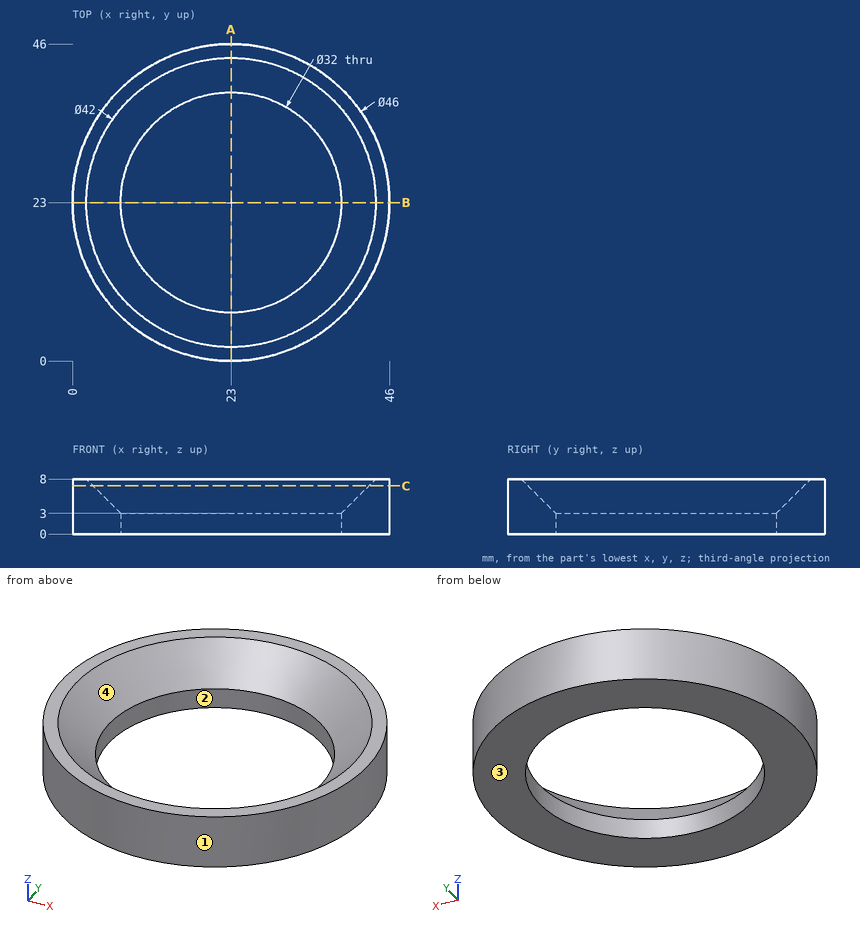
Part print with two shaded views. Sizes in mm from the minimum x, y, z corner. Coordinates: 2 decimals unless noted, no trailing zeros. Write each loop counter-clockwise with the first axis right and the second up, starting at its lowest first coordinate (ties: lowest second). Pieces come first, ordered by that corner, then holes. Notation, with made-up numbers: (58, 22) -> (62, 22) arc R20 cw to (62, 48) -> close; hole circle Ø3 at (89, -11.75). An arc over 180 degrees is marked (long way). Return JSON: item names as keys, results as strings. Group by question number.
Q1. Pull direction Y, two halves, no side cores. Call the marked faces 1, 2, 3 and 4: released by +Y, released by -Y, zero draft, split by the parting line, or undercut.
Q2. Cut at C-C, the plane z = 7. Give the cut face in (x, y).
Q3. Cut at A-A, the plane x = 23. Give the cut face in (y, z), then the cut area to 3 significant figures.
Q4. Flat gauge pins, fed straight in: pin 1 (5 mm diameter, centred on x = 37, y = 14, fed in from -Z); pin 2 (2 mm diameter, centred on x = 27, z = 5.5, fed in from -Y); pin 3 (3 mm diameter, centred on y = 25, z = 4, fed in from -X); pin 4 (3 mm diameter, centred on x = 20, z = 7, fed in from -Y). Where does each tip first touch, or does it go through?
Q5. Drill centre lines: line 1 (X direction, y = 23, z = 0.9); line 2 (X direction, y = 19.5, z = 3.25). Where is each one in solid material? Low to high.
Returned:
{
 "1": {"face 1": "split by the parting line", "face 2": "undercut", "face 3": "zero draft", "face 4": "undercut"},
 "2": {"outline": "circle Ø46 at (23, 23); hole circle Ø40 at (23, 23)"},
 "3": {"outline": "(0, 0) -> (7, 0) -> (7, 3) -> (2, 8) -> (0, 8) -> close; (39, 0) -> (46, 0) -> (46, 8) -> (44, 8) -> (39, 3) -> close", "area": "87.0 mm2"},
 "4": {"pin 1": "stops at z = 0", "pin 2": "stops at y = 0.2", "pin 3": "stops at x = 0.01", "pin 4": "stops at y = 0.05"},
 "5": {"line 1": "x = 0 to 7, 39 to 46", "line 2": "x = 0.27 to 7.13, 38.87 to 45.73"}
}
